Read the model definition and answer for the solid it produces. Units are mm, in the model's axes. Give positions to 0.01 mm unless a question says otherwise; leave off trailing zeros. Order: outer loops, then holes, each group sorted by start corner. A loop starts at its lowest first (then second) coordinate and runs counter-clockwise, first axis right, second up.
```python
from build123d import *

# Parameters (mm, degrees)
SKETCH1_R               = 6.35
BASIC_ROD_DEPTH         = 27.70251
BASIC_ROD_DEPTH_BACK    = 27.70251
THEX_DEPTH              = 27.70251
SKETCH2_R               = 4
INTERNAL_CUT_DEPTH      = 28.70251
INTERNAL_CUT_DEPTH_BACK = 28.70251


with BuildPart() as part:
    # Sketch1 → Basic Rod (new body, two sides)
    with BuildSketch(Plane.XY) as basic_rod_sk:
        Circle(SKETCH1_R)
    extrude(amount=BASIC_ROD_DEPTH)
    extrude(basic_rod_sk.sketch, amount=-BASIC_ROD_DEPTH_BACK)

    # Sketch8 → THex (add, symmetric)
    with BuildSketch(Plane.XY):
        with BuildLine():
            Line((-0.888411378, 6.819423871), (-5.461588622, 4.179098758))
            ThreePointArc((-5.461588622, 4.179098758), (-5.955700003, 3.438525), (-6.35, 2.640325113))
            Line((-6.35, 2.640325113), (-6.35, -2.640325113))
            ThreePointArc((-6.35, -2.640325113), (-5.955700003, -3.438525), (-5.461588622, -4.179098758))
            Line((-5.461588622, -4.179098758), (-0.888411378, -6.819423871))
            ThreePointArc((-0.888411378, -6.819423871), (0, -6.87705), (0.888411378, -6.819423871))
            Line((0.888411378, -6.819423871), (5.461588622, -4.179098758))
            ThreePointArc((5.461588622, -4.179098758), (5.955700003, -3.438525), (6.35, -2.640325113))
            Line((6.35, -2.640325113), (6.35, 2.640325113))
            ThreePointArc((6.35, 2.640325113), (5.955700003, 3.438525), (5.461588622, 4.179098758))
            Line((5.461588622, 4.179098758), (0.888411378, 6.819423871))
            ThreePointArc((0.888411378, 6.819423871), (0, 6.87705), (-0.888411378, 6.819423871))
        make_face()
    extrude(amount=THEX_DEPTH, both=True)

    # Sketch2 → Internal Cut (cut, two sides)
    with BuildSketch(Plane.XY) as internal_cut_sk:
        Circle(SKETCH2_R)
    extrude(amount=INTERNAL_CUT_DEPTH, mode=Mode.SUBTRACT)
    extrude(internal_cut_sk.sketch, amount=-INTERNAL_CUT_DEPTH_BACK, mode=Mode.SUBTRACT)


solid = part.part
```
1) The part is cut by section B-B on x = 0. Determine the outline of the cut face in (y, z).
Final values:
outline: (-6.88, -27.7) - (-4, -27.7) - (-4, 27.7) - (-6.88, 27.7) - close; (4, -27.7) - (6.88, -27.7) - (6.88, 27.7) - (4, 27.7) - close
2) The part is cut by section A-A on y = 0. Determine the outline of the cut face in (x, z), and give its area (3 significant figures).
Final values:
outline: (-6.35, -27.7) - (-4, -27.7) - (-4, 27.7) - (-6.35, 27.7) - close; (4, -27.7) - (6.35, -27.7) - (6.35, 27.7) - (4, 27.7) - close
area: 260 mm2
3) For a pull along Y with two mould halves and no side action, classify faces 1 (the face through (-0.867, -3.905, 0.388)), 2 (the face through (-3.21, -5.48, 0.39)), 3 (the face through (-5.95, 3.45, 0.39)) as released by +Y, released by -Y, zero draft, split by the parting line, or undercut.
Final values:
face 1: undercut
face 2: released by -Y
face 3: released by +Y
4) The part is cut by section C-C on y = -6. Determine the outline of the cut face in (x, z).
Final values:
outline: (-2.31, -27.7) - (2.31, -27.7) - (2.31, 27.7) - (-2.31, 27.7) - close
5) Consider L1, parallel to X at y = 0, z = 9; L2, parallel to Y at x = 0, z = 10; L3, parallel to X at y = -1, z = 17. Determine where each line is inside the solid, lowest interval first.
Final values:
L1: x = -6.35 to -4, 4 to 6.35
L2: y = -6.88 to -4, 4 to 6.88
L3: x = -6.35 to -3.87, 3.87 to 6.35
6) Given pin 1 (2 mm diameter, centred on y = 5, z = -21, fed in from +X); pin 2 (1 mm diameter, centred on x = 3, z = 14.5, fed in from +Y); pin 3 (6 mm diameter, centred on x = 4, z = -1.5, fed in from -Y) (3 decimals), each flat-ended and moving along its own axis, determine where each tip first touches the part or whether it passes through.
Final values:
pin 1: stops at x = 5.59
pin 2: stops at y = 5.89
pin 3: stops at y = -6.755
